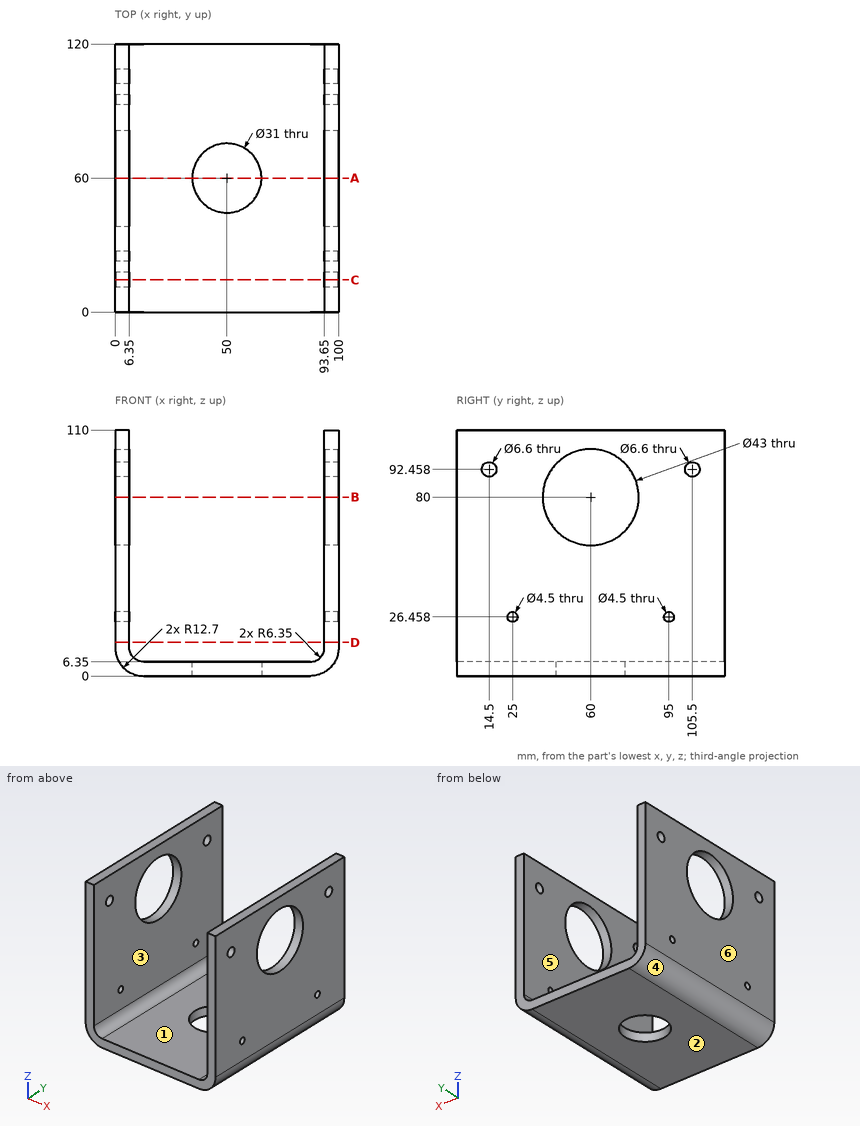
The figure shows three views and two pictorial views of one solid part (mm, origin at its lowest corner). Answer the questions. A direction names the side the tool comes from. Round coordinates to 2 decimals unless told otherwise and drop trailing zeros. Order: outer loops, then holes, each group sorted by start corner. A loop starts at its lowest first (then second) coordinate and runs counter-clockwise, first axis right, second up. Notation, with made-up numbers: M 32.25,88.25 L 89.25,88.25 A17 cw 89.25,97.25 Z; hole C 76.25,42 d1. An arc over 180 degrees is marked long. Put each result on its own line as item: value. Start each with the question number.
Q1. For a pull along X with two mould halves and no side action, classify the marked faces 1, 2, 3 and 4 as pulls with the +X half, pulls with the -X half, needs draft (parallel to the pull), parting line crosses it, or undercut.
Q2. Straight lines are drawn through the part: L1, parallel to X at y = 115, z = 51.5; L2, parallel to Y at x = 96, z = 80; L3, parallel to X at y = 27, z = 8. For each, find the intervals that lie inside material, in ascending order. Write a range as [from, to].
Q3. Flat-ended cylindrical pins translate along their axes: pin 1 (4 mm diameter, centred on y = 25, z = 26.458, fed in from +X); pin 2 (10 mm diameter, centred on x = 80, y = 43, fed in from +Z). Find the tip coordinate at first contact, or state that the pin passes through.
Q4. Section D-D, the plane z = 15 is taken. Write down the section's boundary in (x, y), and give its area (3 significant figures).
Q5. Section A-A, the plane y = 60 is taken. Write down the section's boundary in (x, z), and give its area (3 significant figures).
Q6. Section B-B, the plane z = 80 is taken. Write down the section's boundary in (x, y).
Q7. Section C-C, the plane y = 14.5 is taken. Write down the section's boundary in (x, z).
Q8. A tool of negligible diameter and unlimited length cuts with its end or side. For the marked faces 5 and 6, from which of +Z, -Z, +X, -X, +Y, -Y can it reach the whole face along a straight path? Write none if from no direction.
Findings below:
1. face 1: undercut
1. face 2: needs draft
1. face 3: undercut
1. face 4: pulls with the -X half
2. L1: x = [0, 6.35], [93.65, 100]
2. L2: y = [0, 38.5], [81.5, 120]
2. L3: x = [0.9, 8.43], [91.57, 99.1]
3. pin 1: passes through
3. pin 2: stops at z = 6.35
4. outline: M 0,0 L 6.35,0 L 6.35,120 L 0,120 Z; M 93.65,0 L 100,0 L 100,120 L 93.65,120 Z
4. area: 1,520 mm^2
5. outline: M 0,12.7 A12.7 ccw 12.7,0 L 34.5,0 L 34.5,6.35 L 12.7,6.35 A6.35 cw 6.35,12.7 L 6.35,58.5 L 0,58.5 Z; M 0,101.5 L 6.35,101.5 L 6.35,110 L 0,110 Z; M 65.5,0 L 87.3,0 A12.7 ccw 100,12.7 L 100,58.5 L 93.65,58.5 L 93.65,12.7 A6.35 cw 87.3,6.35 L 65.5,6.35 Z; M 93.65,101.5 L 100,101.5 L 100,110 L 93.65,110 Z
5. area: 1,160 mm^2
6. outline: M 0,0 L 6.35,0 L 6.35,38.5 L 0,38.5 Z; M 0,81.5 L 6.35,81.5 L 6.35,120 L 0,120 Z; M 93.65,0 L 100,0 L 100,38.5 L 93.65,38.5 Z; M 93.65,81.5 L 100,81.5 L 100,120 L 93.65,120 Z
7. outline: M 0,12.7 A12.7 ccw 12.7,0 L 87.3,0 A12.7 ccw 100,12.7 L 100,89.16 L 93.65,89.16 L 93.65,12.7 A6.35 cw 87.3,6.35 L 12.7,6.35 A6.35 cw 6.35,12.7 L 6.35,89.16 L 0,89.16 Z; M 0,95.76 L 6.35,95.76 L 6.35,110 L 0,110 Z; M 93.65,95.76 L 100,95.76 L 100,110 L 93.65,110 Z
8. face 5: +Z, +Y, -Y
8. face 6: +Z, -Z, -X, +Y, -Y
